Verification items for the finished model (mm, model axes). A direction names the side the tool comes from. Coordinates: 2 decimals unless noted, no trailing zeros. Write each loop counter-clockwise with the first axis right and the second up, starting at its lowest first coordinate (ties: lowest second). Pieces come first, ordered by that corner, then holes. Notation, with made-up numbers: (82, 43.5) -> (117, 43.5) arc R19 ccw to (117, 77.5) -> close; hole circle Ø4 at (67.25, 78). An arc over 180 degrees is marked (long way). Answer in a Markdown table with one row per item.
```python
from build123d import *

# Parameters (mm, degrees)
SKETCH_W         = 89.59788
SKETCH_H         = 20
PAD_DEPTH        = 10
SKETCH001_W      = 4
SKETCH001_H      = 19
PAD001_DEPTH     = 3
HOLE_D           = 5.5
HOLE_DEPTH       = 25
HOLE_CBORE_D     = 10
HOLE_CBORE_DEPTH = 4
FILLET_R         = 2


with BuildPart() as part:
    # Sketch (on Face2 of Binder) → Pad (new body)
    with BuildSketch(Plane.YZ.offset(237.459106)):
        with Locations((0.426081, 189.84877)):
            Rectangle(SKETCH_W, SKETCH_H)
        with BuildLine():
            ThreePointArc((-16.372859, 192.857809), (-19.372859, 189.857809), (-16.372859, 186.857809))
            Line((-16.372859, 186.857809), (17.225021, 186.857809))
            ThreePointArc((17.225021, 186.857809), (20.225021, 189.857809), (17.225021, 192.857809))
            Line((-16.372859, 192.857809), (17.225021, 192.857809))
        make_face(mode=Mode.SUBTRACT)
    extrude(amount=PAD_DEPTH)

    # Sketch001 (on Face9 of Pad) → Pad001 (join)
    with BuildSketch(Plane(origin=(237.459106, 0, 0), x_dir=(0, -1, 0), z_dir=(-1, 0, 0))):
        with Locations((-23.225021, 189.84877)):
            Rectangle(SKETCH001_W, SKETCH001_H)
        with Locations((22.372859, 189.857809)):
            Rectangle(SKETCH001_W, SKETCH001_H)
    extrude(amount=PAD001_DEPTH)

    # Hole
    with Locations(Plane.YZ.offset(247.459106)):
        with Locations((-34.372859, 189.857809), (35.225021, 189.84877)):
            CounterBoreHole(HOLE_D / 2, HOLE_CBORE_D / 2, HOLE_CBORE_DEPTH, depth=HOLE_DEPTH)

    # Fillet
    fillet_edges = [part.edges().sort_by_distance(p)[0] for p in [
        (242.459106, 45.225021, 199.84877),
        (242.459106, 45.225021, 179.84877),
        (242.459106, -44.372859, 199.84877),
        (242.459106, -44.372859, 179.84877),
    ]]
    fillet(fillet_edges, radius=FILLET_R)


with BuildPart() as part_1:
    # Body placement: moved
    add(part.part.moved(Location((-253.7, 0, -183.9))))


solid = part_1.part
```
1. Section check D-D, the plane z = 4.5. State how many separate pieces and enclosed holes the cut face has, plus the area to 3 significant figures.
Geometry says:
| item | result |
|---|---|
| separate pieces | 4 |
| enclosed holes | 0 |
| area | 399 mm^2 |
2. Thickness scan on line 1 (Z direction, x = -9.75, y = 17); line 2 (Y direction, x = -16.5, z = 5.25); line 3 (Y direction, x = -14.75, z = 5.5). Record the ranges inside material, lowest first. Write a range as from..to.
Geometry says:
| item | result |
|---|---|
| line 1 | -4.05..2.96, 8.96..15.95 |
| line 2 | -24.37..-20.37, 21.23..25.23 |
| line 3 | -44.37..-37.08, -31.66..-19.34, 20.19..32.51, 37.94..45.23 |
3. Section check B-B, the plane x = -18.25. Record the boundary of the cut face in (y, z), plus the area to 3 significant figures.
Geometry says:
| item | result |
|---|---|
| outline | (-24.37, -3.54) -> (-20.37, -3.54) -> (-20.37, 15.46) -> (-24.37, 15.46) -> close; (21.23, -3.55) -> (25.23, -3.55) -> (25.23, 15.45) -> (21.23, 15.45) -> close |
| area | 152 mm^2 |
4. Section check A-A, the plane y = 0. Record the boundary of the cut face in (x, z), plus the area to 3 significant figures.
Geometry says:
| item | result |
|---|---|
| outline | (-16.24, -4.05) -> (-6.24, -4.05) -> (-6.24, 2.96) -> (-16.24, 2.96) -> close; (-16.24, 8.96) -> (-6.24, 8.96) -> (-6.24, 15.95) -> (-16.24, 15.95) -> close |
| area | 140 mm^2 |
5. Depth check by flat-ended pin: P1, Ø5, axis at y = 35.23, z = 5.95, coming from the +X side; P2, Ø0.9, axis at x = -18.5, y = 23, coming from the +Z side; P3, Ø12, axis at y = 34.5, z = -1.5, coming from the -X side; P4, Ø2.5, axis at x = -18.5, z = 6.5, coming from the +Y side (3 decimals). Enter the tip coordinate at first touch or a pass-through.
Geometry says:
| item | result |
|---|---|
| P1 | through |
| P2 | z = 15.45 |
| P3 | x = -16.24 |
| P4 | y = 25.225 |
6. Section check C-C, the plane z = -0.5. Record the boundary of the cut face in (x, y).
Geometry says:
| item | result |
|---|---|
| outline | (-19.24, -24.37) -> (-16.24, -24.37) -> (-16.24, -44.37) -> (-6.24, -44.37) -> (-6.24, 45.23) -> (-16.24, 45.23) -> (-16.24, 25.23) -> (-19.24, 25.23) -> (-19.24, 21.23) -> (-16.24, 21.23) -> (-16.24, -20.37) -> (-19.24, -20.37) -> close |
7. Tool access check on faces 1 (the flat face through (-18, 23, 15.449)), 2 (the flat face through (-18, -22, -3.542)), 3 (the flat face through (-11, 0, 8.958)), 4 (the flat face through (-10.241, 37.4, 3.8)). Record the directions out of +Z, -Z, +X, -X, +Y, -Y that give a thin tool (end or side, any length) a straight path to the whole face; none if there is none.
Geometry says:
| item | result |
|---|---|
| face 1 | +Z, -X, +Y, -Y |
| face 2 | -Z, -X, +Y, -Y |
| face 3 | +X, -X |
| face 4 | +X |
8. Mould release check, pull along Y, two halves, no side actions. Record for faces 5 (the flat face through (-11, 45.225, 6)), 6 (the cylindrical face through (-13.283, -31.626, 6.079)), 7 (the flat face through (-11, 0, 15.949)): released by +Y, released by -Y, zero draft, split by the parting line, or undercut.
Geometry says:
| item | result |
|---|---|
| face 5 | released by +Y |
| face 6 | undercut |
| face 7 | zero draft |
